Print and shaded views of the part. All mm, measured from the part's lowest x, y and z. Coordinates: 2 decimals unless noted, no trailing zeros. Order: outer loops, then holes, each group sorted by start corner. A loop starts at its lowest first (then second) coordinate and runs counter-clockwise, first axis right, second up. Notation, with made-up numbers: M 53,81 L 81,81 A19 ccw 81,94 Z; hole C 18,6 d4. An arc over 180 degrees is marked long. Use a Markdown table: item, result. Add a question column.
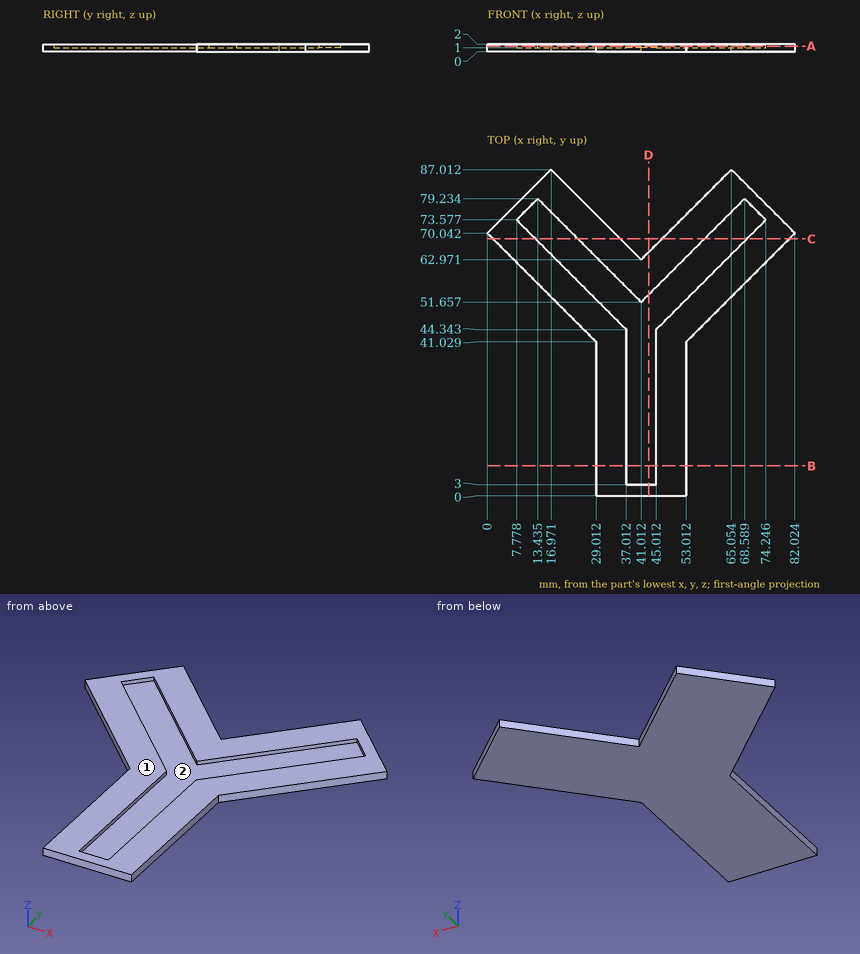
(1) Slice it at D-D on x = 43. Give the cut face in (y, z) (1 decimal).
(2) Slice it at B-B on y = 8. Give the cut face in (x, z), and give its area (3 significant figures).
(3) Slice it at A-A on z = 1.45. Give the cut face in (x, y) (1 decimal), and give its area (3 significant figures).
(4) Slice it at C-C on y = 68.5. Give the cut face in (x, z) (1 decimal), and give its area (3 significant figures).
(5) Mould opens along X. For the marked faces 1 and 2 say: released by +X, released by -X, zero draft, split by the parting line, or undercut.
(6) Drill centre lines: line 1 along X through (y, z) = (55, 1.4) (1 decimal); line 2 along X through (y, z) = (62, 1.5) (1 decimal); line 3 along Z through (x, y) = (10.5, 76). Where is each one in solid material? Low to high. Write a range as from..to.
(7) Drop flat-ended pins along their axis: P1, Ø0.6, axis at y = 11.5, z = 1, coming from the +X side; P2, Ø1.1, axis at y = 30.5, z = 1.5, coming from the -X side. Give the stop position or say it passes through.
Solutions:
| question | item | result |
|---|---|---|
| 1 | outline | M 0,0 L 65,0 L 65,2 L 53.6,2 L 53.6,1 L 3,1 L 3,2 L 0,2 Z |
| 2 | outline | M 29.01,0 L 53.01,0 L 53.01,2 L 45.01,2 L 45.01,1 L 37.01,1 L 37.01,2 L 29.01,2 Z |
| 2 | area | 40.0 mm² |
| 3 | outline | M 0,70 L 29,41 L 29,0 L 53,0 L 53,41 L 82,70 L 65.1,87 L 41,63 L 17,87 Z; hole M 7.8,73.6 L 37,44.3 L 37,3 L 45,3 L 45,44.3 L 74.2,73.6 L 68.6,79.2 L 41,51.7 L 13.4,79.2 Z |
| 3 | area | 2,050 mm² |
| 4 | outline | M 1.5,0 L 35.5,0 L 35.5,2 L 24.2,2 L 24.2,1 L 12.9,1 L 12.9,2 L 1.5,2 Z; M 46.5,0 L 80.5,0 L 80.5,2 L 69.2,2 L 69.2,1 L 57.9,1 L 57.9,2 L 46.5,2 Z |
| 4 | area | 113 mm² |
| 5 | face 1 | zero draft |
| 5 | face 2 | undercut |
| 6 | line 1 | 15..26.4, 37.7..44.4, 55.7..67 |
| 6 | line 2 | 8..19.4, 30.7..51.4, 62.7..74 |
| 6 | line 3 | 0..1 |
| 7 | P1 | x = 53.01 |
| 7 | P2 | x = 29.01 |
